```python
from build123d import *

# Parameters (mm, degrees)
F3_DEPTH = 4


with BuildPart() as f1:
    # F0 (on Front) → F1 (revolve)
    with BuildSketch(Plane.XZ):
        Polygon((0, 2.5), (0, 0), (17, 0), (17, 4.25), (12, 4.25), (12, 2.5), align=None)
    revolve(axis=Axis((8.5, 0, 0), (-1, 0, 0)))

    # F2 (on face) → F3 (cut)
    with BuildSketch(Plane.YZ.offset(17)):
        Polygon((1.154701, 2), (-1.154701, 2), (-2.309401, 0), (-1.154701, -2), (1.154701, -2), (2.309401, 0), align=None)
    extrude(amount=-F3_DEPTH, mode=Mode.SUBTRACT)


solid = f1.part
```
Could you check a few things on this model? Use its own coordinates, in mm. A direction names the side the tool comes from. Round coordinates to 2 decimals unless told otherwise and drop trailing zeros. Write each loop counter-clockwise with the first axis right and the second up, starting at its lowest first coordinate (ties: lowest second). Pieces come first, ordered by that corner, then holes.
(1) For pin 1 (1 mm diameter, centred on x = 5.5, z = 1, fed in from -Y); pin 2 (5 mm diameter, centred on x = 2.5, y = -3, fed in from -Z); pin 3 (4 mm diameter, centred on x = 5.5, z = 3, fed in from -Y), each with a flat end and sliding along its axis, tell me the tip position at first contact or that it passes through.
Findings below:
pin 1: stops at y = -2.45
pin 2: stops at z = -2.45
pin 3: stops at y = -2.29
(2) Thinking about a two-plate mould opening in Z: for faces 4 (the face through (15.03, -1.74, -0.99)), 5 (the face through (5.92, -2.44, -0.54)), 6 (the face through (0, 0, 0)), which applies, +Z half, -Z half, draft (parallel to the pull), parting line (faces both ways), or undercut?
Findings below:
face 4: undercut
face 5: parting line
face 6: draft
(3) Suppose I cut it at C-C on x = 4. Write out the boundary of the cut face in (y, z), and give its area (3 significant figures).
Findings below:
outline: circle Ø5 at (0, 0)
area: 19.6 mm2
(4) Which directions (+Z, -Z, +X, -X, +Y, -Y) give clear straight access to the entire face, cutting with the end or side of a thin tool? Please do faces 1 (the face through (12, -2, 2)), 2 (the face through (14.465, 3.584, 2.285)), 3 (the face through (15.03, 1.74, 0.99)).
Findings below:
face 1: -X
face 2: +X, -X
face 3: +X
(5) Suppose I cut it at A-A on y = 0. Write out the boundary of the cut face in (x, z).
Findings below:
outline: (0, -2.5) - (12, -2.5) - (12, -4.25) - (17, -4.25) - (17, -2) - (13, -2) - (13, 2) - (17, 2) - (17, 4.25) - (12, 4.25) - (12, 2.5) - (0, 2.5) - close
(6) Suppose I cut it at D-D on z = 3.75. Write out the boundary of the cut face in (x, y), and give its area (3 significant figures).
Findings below:
outline: (12, -2) - (17, -2) - (17, 2) - (12, 2) - close
area: 20.0 mm2
(7) Suppose I cut it at B-B on z = 0.5. Write out the boundary of the cut face in (x, y).
Findings below:
outline: (0, -2.45) - (12, -2.45) - (12, -4.22) - (17, -4.22) - (17, -2.02) - (13, -2.02) - (13, 2.02) - (17, 2.02) - (17, 4.22) - (12, 4.22) - (12, 2.45) - (0, 2.45) - close
(8) If I drill on probe 1 along X at (y, z) = (-0.5, 0); probe 2 along Z at (x, y) = (13.25, -0.25); probe 3 along X at (y, z) = (-3.25, 2), over which ranges is the centre line in solid material (lowest first)?
Findings below:
probe 1: x = 0 to 13
probe 2: z = -4.24 to -2, 2 to 4.24
probe 3: x = 12 to 17
